Read the model definition and answer for the solid it produces. Units are mm, in the model's axes. Coordinates: 2 decimals unless noted, no trailing zeros. Order: outer loops, then holes, each group sorted by start corner. A loop starts at its lowest first (then second) coordinate and runs counter-clockwise, first axis right, second up. Notation, with made-up numbers: (-4, 64) - (23, 64) arc R11 ccw to (23, 70) - close; hole circle Ø5 at (-10.5, 29.25). An arc over 180 degrees is marked (long way). Answer as a JSON object with one key per item and string values. Group by question number.
from build123d import *

# Parameters (mm, degrees)
SKETCH1_W           = 10.62
SKETCH1_H           = 6.3
BOSS_EXTRUDE1_DEPTH = 8.8
SKETCH2_W           = 0.8
SKETCH2_H           = 0.5
BOSS_EXTRUDE2_DEPTH = 3.2
CUT_EXTRUDE1_REACH  = 12.62
SKETCH4_W           = 2
SKETCH4_H           = 4
CUT_EXTRUDE2_DEPTH  = 3.15
CUT_EXTRUDE2_TAPER  = 10


with BuildPart() as part:
    # Sketch1 → Boss-Extrude1 (new body)
    with BuildSketch(Plane(origin=(0, 0, 0), x_dir=(1, 0, 0), z_dir=(0, 1, 0))):
        Rectangle(SKETCH1_W, SKETCH1_H)
    extrude(amount=BOSS_EXTRUDE1_DEPTH)

    # Sketch2 → Boss-Extrude2 (add)
    with BuildSketch(Plane(origin=(0, 0, 0), x_dir=(1, 0, 0), z_dir=(0, 1, 0))):
        with Locations((1.27, 0.2)):
            Rectangle(SKETCH2_W, SKETCH2_H)
        with Locations((3.81, 0.2)):
            Rectangle(SKETCH2_W, SKETCH2_H)
        with Locations((-1.27, 0.2)):
            Rectangle(SKETCH2_W, SKETCH2_H)
        with Locations((-3.81, 0.2)):
            Rectangle(SKETCH2_W, SKETCH2_H)
    extrude(amount=-BOSS_EXTRUDE2_DEPTH)

    # Sketch3 → Cut-Extrude1 (cut, up to next)
    with BuildSketch(Plane(origin=(5.31, 0, 0), x_dir=(0, 0, -1), z_dir=(1, 0, 0)), mode=Mode.PRIVATE) as cut_extrude1_sk1:
        with BuildLine():
            ThreePointArc((-3.15, 4.7), (-2.974264069, 5.124264069), (-2.55, 5.3))
            Line((-2.55, 5.3), (-2.337822174, 5.3))
            Line((-2.337822174, 5.3), (-1.4, 8.8))
            Line((-1.4, 8.8), (-3.15, 8.8))
            Line((-3.15, 8.8), (-3.15, 4.7))
        make_face()
    cut_extrude1_tool1 = extrude(cut_extrude1_sk1.sketch, amount=-CUT_EXTRUDE1_REACH, mode=Mode.PRIVATE) & part.part
    add(cut_extrude1_tool1.solids().sort_by_distance((5.31, 7.227986, 2.489914))[0], mode=Mode.SUBTRACT)
    # Sketch3 → Cut-Extrude1 (cut, up to next)
    with BuildSketch(Plane(origin=(5.31, 0, 0), x_dir=(0, 0, -1), z_dir=(1, 0, 0)), mode=Mode.PRIVATE) as cut_extrude1_sk2:
        Polygon((3.15, 8.8), (1.4, 8.8), (3.15, 2.268911087), align=None)
    cut_extrude1_tool2 = extrude(cut_extrude1_sk2.sketch, amount=-CUT_EXTRUDE1_REACH, mode=Mode.PRIVATE) & part.part
    add(cut_extrude1_tool2.solids().sort_by_distance((5.31, 6.62297, -2.566667))[0], mode=Mode.SUBTRACT)

    # Sketch4 → Cut-Extrude2 (cut)
    with BuildSketch(Plane.XY.offset(3.15)):
        with Locations((-3.81, 2.268911087)):
            Rectangle(SKETCH4_W, SKETCH4_H)
        with Locations((-1.27, 2.268911087)):
            Rectangle(SKETCH4_W, SKETCH4_H)
        with Locations((1.27, 2.268911087)):
            Rectangle(SKETCH4_W, SKETCH4_H)
        with Locations((3.81, 2.268911087)):
            Rectangle(SKETCH4_W, SKETCH4_H)
    extrude(amount=-CUT_EXTRUDE2_DEPTH, taper=CUT_EXTRUDE2_TAPER, mode=Mode.SUBTRACT)


solid = part.part
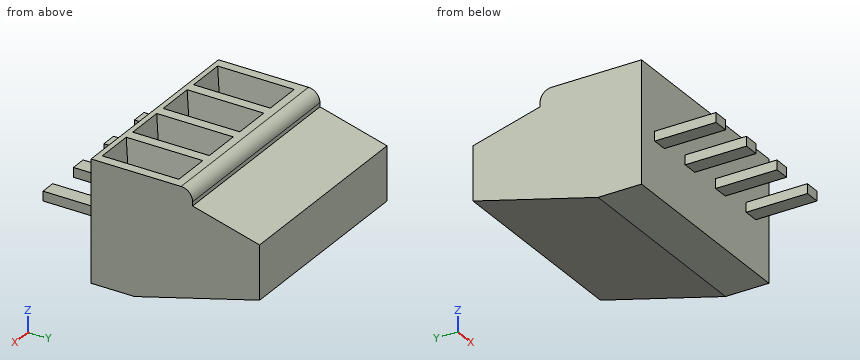
1. Straight lines are drawn through the part: L1, parallel to Y at x = -2.75, z = -0.25; L2, parallel to Y at x = 4, z = 1.25; L3, parallel to Z at x = -1.75, y = 7. For each, find the intervals that lie inside material, in ascending order.
2. A cutting plane is placed at B-B on z = -0.25. Write down the section's boundary in (x, y).
3. A cutting plane is placed at C-C on x = 0. Write down the section's boundary in (y, z), and give its area (3 significant figures).
4. A cutting plane is placed at D-D on z = 1. State how many separate pieces and enclosed holes the cut face has, and give its area (3 significant figures).
5. A cutting plane is placed at A-A on y = -1.5. Write down the section's boundary in (x, z).
6. Given pin 1 (0.9 mm diameter, centred on x = -1, y = -1, fed in from -Z); pin 2 (0.6 mm diameter, centred on y = -1.5, z = -0.5, fed in from -X); pin 3 (3 mm diameter, centred on x = -1.5, y = 3, fed in from -Z), each flat-ended and moving along its own axis, determine where each tip first touches the part or whether it passes through.
Derived:
{
 "1": {"L1": "y = 0 to 8.8", "L2": "y = 0 to 0.6, 3.93 to 8.8", "L3": "z = -1.88 to 1.88"},
 "2": {"outline": "(-5.31, 0) - (-4.21, 0) - (-4.21, -3.2) - (-3.41, -3.2) - (-3.41, 0) - (-1.67, 0) - (-1.67, -3.2) - (-0.87, -3.2) - (-0.87, 0) - (0.87, 0) - (0.87, -3.2) - (1.67, -3.2) - (1.67, 0) - (3.41, 0) - (3.41, -3.2) - (4.21, -3.2) - (4.21, 0) - (5.31, 0) - (5.31, 8.8) - (-5.31, 8.8) - close"},
 "3": {"outline": "(0, -3.15) - (2.27, -3.15) - (8.8, -1.4) - (8.8, 1.4) - (5.3, 2.34) - (5.3, 2.55) arc R0.6 ccw to (4.7, 3.15) - (0, 3.15) - close", "area": "45.2 mm2"},
 "4": {"separate pieces": "1", "enclosed holes": "4", "area": "77.4 mm2"},
 "5": {"outline": "(-4.21, -0.45) - (-3.41, -0.45) - (-3.41, 0.05) - (-4.21, 0.05) - close; (-1.67, -0.45) - (-0.87, -0.45) - (-0.87, 0.05) - (-1.67, 0.05) - close; (0.87, -0.45) - (1.67, -0.45) - (1.67, 0.05) - (0.87, 0.05) - close; (3.41, -0.45) - (4.21, -0.45) - (4.21, 0.05) - (3.41, 0.05) - close"},
 "6": {"pin 1": "stops at z = -0.45", "pin 2": "stops at x = -4.21", "pin 3": "stops at z = -3.15"}
}
